Autodesk Inventor part; units mm, degrees
ref_plane "YZ Plane" through (0, 0, 0) normal (1, 0, 0) x (0, 1, 0)
ref_plane "XZ Plane" through (0, 0, 0) normal (0, 1, 0) x (-1, 0, 0)
ref_plane "XY Plane" through (0, 0, 0) normal (0, 0, 1) x (1, 0, 0)
sketch "T-Slot 4040 Base" plane through (0, 0, 0) normal (0, 0, 1) x (1, 0, 0)
  line L0 (-28, 0) -> (28, 0) construction
  line L1 (0, -28) -> (0, 28) construction
  circle A0 centre (0, 0) radius 5.1
  line L2 (-7.5, -7.5) -> (7.5, -7.5)
  line L3 (7.5, -7.5) -> (7.5, 7.5)
  line L4 (7.5, 7.5) -> (-7.5, 7.5)
  line L5 (-7.5, 7.5) -> (-7.5, -7.5)
  line L6 (-7.5, -7.5) -> (7.5, 7.5) construction
  line L7 (7.5, -7.5) -> (-7.5, 7.5) construction
  line L8 (-20, 20) -> (20, 20)
  line L9 (20, 20) -> (20, -20)
  line L10 (20, -20) -> (-20, -20)
  line L11 (-20, -20) -> (-20, 20)
  line L12 (-20, 20) -> (20, -20) construction
  line L13 (20, 20) -> (-20, -20) construction
  line L14 (20, 5) -> (14.5, 5)
  line L15 (14.5, 5) -> (14.5, 10)
  line L16 (14.5, 10) -> (12.4749, 10)
  line L17 (12.4749, 10) -> (7.5, 5.0251)
  line L18 (5, 20) -> (5, 14.5)
  line L19 (5, 14.5) -> (10, 14.5)
  line L20 (10, 14.5) -> (10, 12.4749)
  line L21 (10, 12.4749) -> (5.0251, 7.5)
  line L22 (18.5, 18.5) -> (11.5, 18.5)
  line L23 (11.5, 18.5) -> (11.5, 11.5)
  line L24 (11.5, 11.5) -> (18.5, 11.5)
  line L25 (18.5, 11.5) -> (18.5, 18.5)
  line L26 (18.5, 18.5) -> (11.5, 11.5) construction
  line L27 (11.5, 18.5) -> (18.5, 11.5) construction
  line L28 (3.0732, 1.3088) -> (4.38, 2.6125) construction
  line L29 (5.905, 4.1338) -> (4.1393, 5.9037)
  line L30 (4.1393, 5.9037) -> (2.6122, 4.3802)
  line L31 (1.3075, 3.0787) -> (3.0732, 1.3088) construction
  line L32 (3.0732, 1.3088) -> (4.1393, 5.9037) construction
  line L33 (5.905, 4.1338) -> (1.3075, 3.0787) construction
  line L34 (4.38, 2.6125) -> (5.905, 4.1338)
  line L35 (2.6122, 4.3802) -> (1.3075, 3.0787) construction
  line L36 (-20, 5) -> (-14.5, 5)
  line L37 (-14.5, 5) -> (-14.5, 10)
  line L38 (-14.5, 10) -> (-12.4749, 10)
  line L39 (-12.4749, 10) -> (-7.5, 5.0251)
  line L40 (-5, 20) -> (-5, 14.5)
  line L41 (-5, 14.5) -> (-10, 14.5)
  line L42 (-10, 14.5) -> (-10, 12.4749)
  line L43 (-10, 12.4749) -> (-5.0251, 7.5)
  line L44 (-18.5, 18.5) -> (-11.5, 18.5)
  line L45 (-11.5, 18.5) -> (-11.5, 11.5)
  line L46 (-11.5, 11.5) -> (-18.5, 11.5)
  line L47 (-18.5, 11.5) -> (-18.5, 18.5)
  line L48 (-5.905, 4.1338) -> (-4.1393, 5.9037)
  line L49 (-4.1393, 5.9037) -> (-2.6122, 4.3802)
  line L50 (-4.38, 2.6125) -> (-5.905, 4.1338)
  line L51 (7.5, -7.5) -> (-7.5, -7.5)
  line L52 (20, -5) -> (14.5, -5)
  line L53 (14.5, -5) -> (14.5, -10)
  line L54 (14.5, -10) -> (12.4749, -10)
  line L55 (12.4749, -10) -> (7.5, -5.0251)
  line L56 (5, -20) -> (5, -14.5)
  line L57 (5, -14.5) -> (10, -14.5)
  line L58 (10, -14.5) -> (10, -12.4749)
  line L59 (10, -12.4749) -> (5.0251, -7.5)
  line L60 (18.5, -18.5) -> (11.5, -18.5)
  line L61 (11.5, -18.5) -> (11.5, -11.5)
  line L62 (11.5, -11.5) -> (18.5, -11.5)
  line L63 (18.5, -11.5) -> (18.5, -18.5)
  line L64 (18.5, -18.5) -> (11.5, -11.5) construction
  line L65 (11.5, -18.5) -> (18.5, -11.5) construction
  line L66 (3.0732, -1.3088) -> (4.38, -2.6125) construction
  line L67 (5.905, -4.1338) -> (4.1393, -5.9037)
  line L68 (4.1393, -5.9037) -> (2.6122, -4.3802)
  line L69 (1.3075, -3.0787) -> (3.0732, -1.3088) construction
  line L70 (3.0732, -1.3088) -> (4.1393, -5.9037) construction
  line L71 (5.905, -4.1338) -> (1.3075, -3.0787) construction
  line L72 (4.38, -2.6125) -> (5.905, -4.1338)
  line L73 (2.6122, -4.3802) -> (1.3075, -3.0787) construction
  line L74 (-4.38, -2.6125) -> (-5.905, -4.1338)
  line L75 (-4.1393, -5.9037) -> (-2.6122, -4.3802)
  line L76 (-5.905, -4.1338) -> (-4.1393, -5.9037)
  line L77 (-12.4749, -10) -> (-7.5, -5.0251)
  line L78 (-10, -12.4749) -> (-5.0251, -7.5)
  line L79 (-10, -14.5) -> (-10, -12.4749)
  line L80 (-5, -14.5) -> (-10, -14.5)
  line L81 (-5, -20) -> (-5, -14.5)
  line L82 (-18.5, -18.5) -> (-11.5, -18.5)
  line L83 (-11.5, -18.5) -> (-11.5, -11.5)
  line L84 (-11.5, -11.5) -> (-18.5, -11.5)
  line L85 (-18.5, -11.5) -> (-18.5, -18.5)
  line L86 (-14.5, -10) -> (-12.4749, -10)
  line L87 (-14.5, -5) -> (-14.5, -10)
  line L88 (-20, -5) -> (-14.5, -5)
  point P0 (15, 15)
  point P1 (3.6062, 3.6062)
  point P2 (3.6062, 3.6062)
  point P3 (15, -15)
  point P4 (3.6062, -3.6062)
  point P5 (3.6062, -3.6062)
  dimension "d9" = 10.2
  dimension "d12" = 40
  dimension "d13" = 40
  dimension "d14" = 5.5
  dimension "d15" = 15
  dimension "d16" = 7
  dimension "d17" = 10
  dimension "d20" = 1.75
  dimension "d21" = 7
  dimension "d22" = 2
  dimension "d29" = 1.5
  dimension "d30" = 2.5
extrude "Extrusion1" add sketch "T-Slot 4040 Base" along normal blind 715 contours L5 L4 L3 L2 | L2 L78 L79 L80 L81 L10 L11 L88 L87 L86 L77 L5 | L2 L3 L55 L54 L53 L52 L9 L10 L56 L57 L58 L59 | L39 L38 L37 L36 L11 L8 L40 L41 L42 L43 L4 L5 | L3 L4 L21 L20 L19 L18 L8 L9 L14 L15 L16 L17
fillet "Rundung1" radius 1 16 edges at (11.5, 18.5, 357.5) (18.5, 18.5, 357.5) (18.5, 11.5, 357.5) (11.5, 11.5, 357.5) (-11.5, 18.5, 357.5) (-18.5, 18.5, 357.5) (-18.5, 11.5, 357.5) (-11.5, 11.5, 357.5) (-18.5, -11.5, 357.5) (-11.5, -11.5, 357.5) (-11.5, -18.5, 357.5) (-18.5, -18.5, 357.5) (11.5, -18.5, 357.5) (11.5, -11.5, 357.5) (18.5, -11.5, 357.5) (18.5, -18.5, 357.5)
fillet "Rundung2" radius 3 4 edges at (20, 20, 357.5) (20, -20, 357.5) (-20, -20, 357.5) (-20, 20, 357.5)
properties part number "T-SLOT 4040 B-Type 715mm"
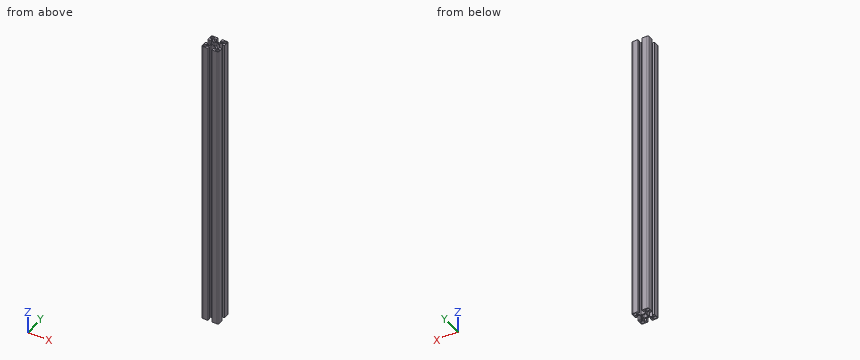
Read the model definition and answer for the solid it produces. Units are mm, in the model's axes. Coordinates: 2 decimals unless noted, no trailing zeros. Write item = value, one per line.
(1) Straight lines are drawn through the part: L1, parallel to Y at x = -14, z = 71.5; L2, parallel to X at y = -17, z = 627.5. For each, find the intervals that lie inside material, in ascending order. Write a range as from..to.
From the geometry:
L1 = -20..-18.5, -11.5..-10, 10..11.5, 18.5..20
L2 = -20..-18.5, -11.5..-5, 5..11.5, 18.5..20
(2) Given pin 1 Ø4 at (x, y) = (5.5, 14) entering from -Z; pin 2 Ø5 at (x, z) = (0.5, 244.5) entering from -Y; pin 3 Ø5 at (x, y) = (11.5, -1.5) entering from -Z, each flat-ended and moving along its own axis, determine where each tip first touches the part or whether it passes through.
From the geometry:
pin_1 = 0
pin_2 = -7.5
pin_3 = through
(3) Section A-A on z = 317 is taken. Count the separate pieces of the cut face and the enclosed holes in it, plus the area to 3 significant figures.
From the geometry:
separate_pieces = 1
enclosed_holes = 5
area = 616 mm2
